Source: CAD feature listing. Evaluate the final solid. Frame: model axes, mm. A direction names the side the tool comes from. Round coordinates to 2 decimals unless told otherwise and drop trailing zeros. Write each loop counter-clockwise with the first axis right and the second up, starting at its lowest first coordinate (ties: lowest second). Pieces come first, ordered by that corner, then holes. Notation, with made-up numbers: M 43.5,-14 L 78.5,-14 A22 ccw 78.5,12 Z; hole C 62,-6.75 d8. An arc over 180 degrees is marked long. Answer in a Markdown table with one row per item.
from build123d import *

# Parameters (mm, degrees)
SKETCH2_R           = 10
BOSS_EXTRUDE1_DEPTH = 3
BOSS_EXTRUDE2_DEPTH = 3
BOSS_EXTRUDE3_DEPTH = 3
BOSS_EXTRUDE7_DEPTH = 2


with BuildPart() as part:
    # Sketch2 → Boss-Extrude1 (new body)
    with BuildSketch(Plane.XY):
        Circle(SKETCH2_R)
    extrude(amount=BOSS_EXTRUDE1_DEPTH)

    # Sketch3 → Boss-Extrude2 (add)
    with BuildSketch(Plane.XY.offset(3)):
        Polygon((-5, -8.660254038), (5, -8.660254038), (5, -33.323330619), (-24.341630951, -57.943882328), (-77.981333294, -57.943882328), (-77.981333294, -47.943882328), (-27.981333294, -47.943882328), (-5, -28.660254038), align=None)
    extrude(amount=-BOSS_EXTRUDE2_DEPTH)

    # Sketch4 → Boss-Extrude3 (add)
    with BuildSketch(Plane.XY.offset(3)):
        with BuildLine():
            Line((-77.981333294, -47.943882328), (-58.662816768, -47.943882328))
            ThreePointArc((-58.662816768, -47.943882328), (-68.322075031, -40.532072779), (-77.981333294, -47.943882328))
        make_face()
    extrude(amount=-BOSS_EXTRUDE3_DEPTH)

    # Sketch5 → Boss-Extrude7 (add)
    with BuildSketch(Plane.XY.offset(3)):
        with BuildLine():
            Line((-3.5, -9.367496998), (-3.5, 9.367496998))
            ThreePointArc((-3.5, 9.367496998), (-9.965563298, 0.829185233), (-5, -8.660254038))
            ThreePointArc((-5, -8.660254038), (-4.264686173, -9.045023596), (-3.5, -9.367496998))
        make_face()
        with BuildLine():
            ThreePointArc((5, -8.660254038), (9.965563298, 0.829185233), (3.5, 9.367496998))
            Line((3.5, 9.367496998), (3.5, -9.367496998))
            ThreePointArc((3.5, -9.367496998), (4.264686173, -9.045023596), (5, -8.660254038))
        make_face()
    extrude(amount=BOSS_EXTRUDE7_DEPTH)


solid = part.part
Q1. Material intervals for probe 1 along X at (y, z) = (-46.5, 1.8); probe 2 along X at (y, z) = (7, 4.4); probe 3 along Z at (x, y) = (2, -3), sorted ascending.
Solutions:
| item | result |
|---|---|
| probe 1 | x = -77.47 to -59.17, -26.26 to -10.7 |
| probe 2 | x = -7.14 to -3.5, 3.5 to 7.14 |
| probe 3 | z = 0 to 3 |
Q2. Access query for faces 4 (the flat face through (5, -21, 2)), 5 (the flat face through (3.5, 0, 4)), 6 (the flat face through (-44, -47.944, 2)), 7 (the flat face through (-16.652, -38.437, 1.521)), 8 (the flat face through (-5, -19, 2)). Directions: +Z, -Z, +X, -X, +Y, -Y. A direction counts if a zero-diameter tool reaches every point of the face in a straight line with its end or side. Return the directions, or none.
Solutions:
| item | result |
|---|---|
| face 4 | +Z, -Z, +X, -Y |
| face 5 | +Z, +Y, -Y |
| face 6 | +Z, -Z, +Y |
| face 7 | +Z, -Z |
| face 8 | +Z, -Z, -X |
Q3. Section C-C (x = -6). Return loops of the section in (y, z), and give its area (3 significant figures).
Solutions:
| item | result |
|---|---|
| outline | M -42.55,0 L -29.5,0 L -29.5,3 L -42.55,3 Z; M -8,0 L 8,0 L 8,5 L -8,5 Z |
| area | 119 mm2 |
Q4. Section D-D (x = -45.5). Return loops of the section in (y, z).
Solutions:
| item | result |
|---|---|
| outline | M -57.94,0 L -47.94,0 L -47.94,3 L -57.94,3 Z |
Q5. Contact query for flat-ended pins moving along their axis: pin 1 Ø0.9 at (y, z) = (-17, 1.5) entering from +X; pin 2 Ø2 at (x, z) = (-21.5, 3) entering from +Y; pin 3 Ø1 at (x, y) = (-65, -40) entering from -Z; pin 4 Ø2 at (y, z) = (-2, 3.5) entering from +X. Output: stop coordinate, or through.
Solutions:
| item | result |
|---|---|
| pin 1 | stops at x = 5 |
| pin 2 | stops at y = -41.67 |
| pin 3 | passes through |
| pin 4 | stops at x = 9.95 |
Q6. Section A-A (z = 1.4). Return loops of the section in (x, y), and give its area (3 significant figures).
Solutions:
| item | result |
|---|---|
| outline | M -77.98,-57.94 L -24.34,-57.94 L 5,-33.32 L 5,-8.66 A10 ccw long -5,-8.66 L -5,-28.66 L -27.98,-47.94 L -58.66,-47.94 A10 ccw -77.98,-47.94 Z |
| area | 1,490 mm2 |
Q7. Pull-direction query (X, two-part tool) for faces 1 (the flat face through (-77.981, -53, 2)), 2 (the flat face through (-51, -57.944, 2)), 3 (the flat face through (-3.5, 0, 4)); classes: pulls with the +X half, pulls with the -X half, needs draft (parallel to the pull), parting line crosses it, or undercut.
Solutions:
| item | result |
|---|---|
| face 1 | pulls with the -X half |
| face 2 | needs draft |
| face 3 | undercut |
Q8. Section B-B (y = 0). Return loops of the section in (x, z), and give its area (3 significant figures).
Solutions:
| item | result |
|---|---|
| outline | M -10,0 L 10,0 L 10,5 L 3.5,5 L 3.5,3 L -3.5,3 L -3.5,5 L -10,5 Z |
| area | 86.0 mm2 |
